from build123d import *

# Parameters (mm, degrees)
SKETCH1_R           = 63.5
SKETCH1_R_2         = 4
BOSS_EXTRUDE1_DEPTH = 5.08
SKETCH2_R           = 69.720778164
SKETCH2_R_2         = 4
BOSS_EXTRUDE2_DEPTH = 5.08
SKETCH4_R           = 1
CUT_EXTRUDE1_DEPTH  = 100.770894631
CUT_EXTRUDE2_DEPTH  = 104.322300355


with BuildPart() as part:
    # Sketch1 → Boss-Extrude1 (new body)
    with BuildSketch(Plane.XY):
        Circle(SKETCH1_R)
        Circle(SKETCH1_R_2, mode=Mode.SUBTRACT)
    extrude(amount=BOSS_EXTRUDE1_DEPTH)

    # Sketch2 → Boss-Extrude2 (add)
    with BuildSketch(Plane.XY.offset(5.08)):
        Circle(SKETCH2_R)
        Circle(SKETCH2_R_2, mode=Mode.SUBTRACT)
    boss_extrude2 = extrude(amount=BOSS_EXTRUDE2_DEPTH)

    # Mirror1: Boss-Extrude2 across plane
    add(boss_extrude2.mirror(Plane(origin=(0, 0, 2.54), x_dir=(1, 0, 0), z_dir=(0, 0, -1))))

    # Sketch4 → Cut-Extrude1 (cut, through all)
    with BuildSketch(Plane(origin=(0, 0, -5.08), x_dir=(-1, 0, 0), z_dir=(0, 0, -1))):
        with Locations((0, 8)):
            Circle(SKETCH4_R)
        with Locations((8, 0)):
            Circle(SKETCH4_R)
        with Locations((0, -8)):
            Circle(SKETCH4_R)
        with Locations((-8, 0)):
            Circle(SKETCH4_R)
    extrude(amount=-CUT_EXTRUDE1_DEPTH, mode=Mode.SUBTRACT)

    # Sketch5 → Revolve1 (revolve)
    with BuildSketch(Plane(origin=(0, 0, 0), x_dir=(0, 0, -1), z_dir=(1, 0, 0)), mode=Mode.PRIVATE) as revolve1_sk:
        with BuildLine():
            Line((-2.54, 63.5), (0, 63.5))
            Line((0, 63.5), (0, 69.720778164))
            ThreePointArc((0, 69.720778164), (-2.54, 72.260778164), (-5.08, 69.720778164))
            Line((-5.08, 69.720778164), (-5.08, 63.5))
            Line((-5.08, 63.5), (-2.54, 63.5))
        make_face()
    revolve(revolve1_sk.sketch.rotate(Axis((0, 0, 5.08), (0, 0, -1)), 90), axis=Axis((0, 0, 5.08), (0, 0, -1)))

    # Sketch6 → Cut-Extrude2 (cut, through all)
    with BuildSketch(Plane(origin=(0, 0, -5.08), x_dir=(-1, 0, 0), z_dir=(0, 0, -1))):
        with BuildLine():
            Line((-7.948419394, -29.571461023), (-13.119997628, -48.811905768))
            ThreePointArc((-13.119997628, -48.811905768), (-15.712841169, -52.016134189), (-19.828493104, -52.242687832))
            ThreePointArc((-19.828493104, -52.242687832), (-39.512451016, -39.512451016), (-52.242687832, -19.828493104))
            ThreePointArc((-52.242687832, -19.828493104), (-52.016134189, -15.712841169), (-48.811905768, -13.119997628))
            Line((-48.811905768, -13.119997628), (-29.571461023, -7.948419394))
            ThreePointArc((-29.571461023, -7.948419394), (-26.086220535, -8.259490359), (-23.628911169, -10.750533731))
            ThreePointArc((-23.628911169, -10.750533731), (-18.356189944, -18.356189944), (-10.750533731, -23.628911169))
            ThreePointArc((-10.750533731, -23.628911169), (-8.259490359, -26.086220535), (-7.948419394, -29.571461023))
        make_face()
        with BuildLine():
            Line((-29.571461023, 7.948419394), (-48.811905768, 13.119997628))
            ThreePointArc((-48.811905768, 13.119997628), (-52.016134189, 15.712841169), (-52.242687832, 19.828493104))
            ThreePointArc((-52.242687832, 19.828493104), (-39.512451016, 39.512451016), (-19.828493104, 52.242687832))
            ThreePointArc((-19.828493104, 52.242687832), (-15.712841169, 52.016134189), (-13.119997628, 48.811905768))
            Line((-13.119997628, 48.811905768), (-7.948419394, 29.571461023))
            ThreePointArc((-7.948419394, 29.571461023), (-8.259490359, 26.086220535), (-10.750533731, 23.628911169))
            ThreePointArc((-10.750533731, 23.628911169), (-18.356189944, 18.356189944), (-23.628911169, 10.750533731))
            ThreePointArc((-23.628911169, 10.750533731), (-26.086220535, 8.259490359), (-29.571461023, 7.948419394))
        make_face()
        with BuildLine():
            ThreePointArc((19.828493104, 52.242687832), (15.712841169, 52.016134189), (13.119997628, 48.811905768))
            Line((13.119997628, 48.811905768), (7.948419394, 29.571461023))
            ThreePointArc((7.948419394, 29.571461023), (8.259490359, 26.086220535), (10.750533731, 23.628911169))
            ThreePointArc((10.750533731, 23.628911169), (14.790224409, 21.334213847), (18.356189944, 18.356189944))
            Line((18.356189944, 18.356189944), (39.512451016, 39.512451016))
            ThreePointArc((39.512451016, 39.512451016), (30.345537475, 46.921380266), (19.828493104, 52.242687832))
        make_face()
        with BuildLine():
            ThreePointArc((52.242687832, 19.828493104), (46.921380266, 30.345537475), (39.512451016, 39.512451016))
            Line((39.512451016, 39.512451016), (18.356189944, 18.356189944))
            ThreePointArc((18.356189944, 18.356189944), (21.334213847, 14.790224409), (23.628911169, 10.750533731))
            ThreePointArc((23.628911169, 10.750533731), (26.086220535, 8.259490359), (29.571461023, 7.948419394))
            Line((29.571461023, 7.948419394), (48.811905768, 13.119997628))
            ThreePointArc((48.811905768, 13.119997628), (52.016134189, 15.712841169), (52.242687832, 19.828493104))
        make_face()
        with BuildLine():
            Line((29.571461023, -7.948419394), (48.811905768, -13.119997628))
            ThreePointArc((48.811905768, -13.119997628), (52.016134189, -15.712841169), (52.242687832, -19.828493104))
            ThreePointArc((52.242687832, -19.828493104), (39.512451016, -39.512451016), (19.828493104, -52.242687832))
            ThreePointArc((19.828493104, -52.242687832), (15.712841169, -52.016134189), (13.119997628, -48.811905768))
            Line((13.119997628, -48.811905768), (7.948419394, -29.571461023))
            ThreePointArc((7.948419394, -29.571461023), (8.259490359, -26.086220535), (10.750533731, -23.628911169))
            ThreePointArc((10.750533731, -23.628911169), (18.356189944, -18.356189944), (23.628911169, -10.750533731))
            ThreePointArc((23.628911169, -10.750533731), (26.086220535, -8.259490359), (29.571461023, -7.948419394))
        make_face()
    extrude(amount=-CUT_EXTRUDE2_DEPTH, mode=Mode.SUBTRACT)


solid = part.part
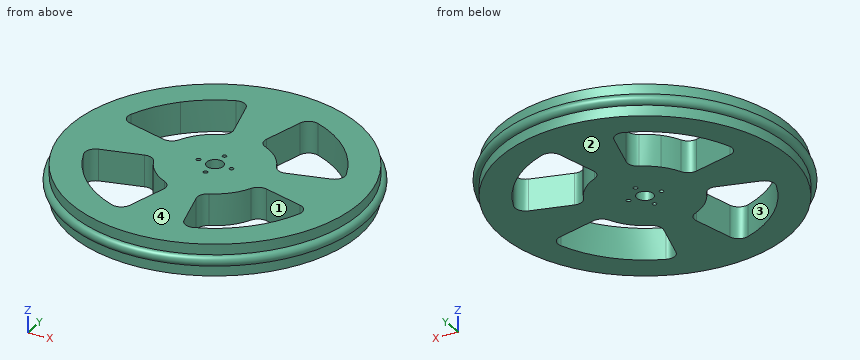
Could you check a few things on this model? Use its own coordinates, in mm. Face numbers are marked on the shaded views. A direction names the side the tool comes from. Give positions to 0.01 mm unless a question says otherwise; leave off trailing zeros.
Item 1: For the marked faces 3 and 4, which set-ups out of +Z, -Z, +X, -X, +Y, -Y let a thin tool reach every point of the face, with its end or its side?
Item 2: I need wall thicknesses on line 1 (Y direction, x = 46, z = 3.25); line 2 (Y direction, x = -16, z = -0.75); line 3 (X direction, y = 34, z = 6.5). Which ranges of each line are inside material? Lowest first, please.
Item 3: If we mould it in two halves opening along X, with no side actions, what happens to the marked faces 1 and 2? For each: pulls with the +X half, pulls with the -X half, needs draft (parallel to the pull), parting line crosses it, or undercut.
Item 4: I'm going to push flat-ended pins straight in: pin 1 (8 mm diameter, centred on x = -43, z = -2.5, fed in from -Y); pin 2 (1.6 mm diameter, centred on x = -8, y = 0, fed in from -Z); pin 3 (5 mm diameter, centred on y = 26.5, z = 0.5, fed in from -X); pin 4 (2 mm diameter, centred on x = 52, y = -50.5, fed in from -Z). Where does each tip first touch, or does it pass through?
Item 5: If we section it at A-A, the plane x = 39: Count the separate pieces of the cut face and the enclosed holes in it, plus the area to 3 significant figures.
Values:
1. face 3: +Z, -Z
1. face 4: +Z, +X, -X, +Y, -Y
2. line 1: y = -55.6 to -31.72, -12.36 to 12.36, 31.72 to 55.6
2. line 2: y = -67.86 to -52.15, -20.44 to 20.44, 52.15 to 67.86
2. line 3: x = -60.87 to -44.34, -9.14 to 9.14, 44.34 to 60.87
3. face 1: undercut
3. face 2: needs draft
4. pin 1: stops at y = -58.85
4. pin 2: passes through
4. pin 3: stops at x = -67.92
4. pin 4: stops at z = 0.71
5. separate pieces: 3
5. enclosed holes: 0
5. area: 886 mm2
